```python
from build123d import *

# Parameters (mm, degrees)
F1_DEPTH = 73.66
F2_R     = 5.08


with BuildPart() as f1:
    # F0 (on Front) → F1 (new body)
    with BuildSketch(Plane.XZ):
        Polygon((-94.9451997876, 22.5552003831), (-94.9451997876, -16.4592005312), (-90.67799896, -16.4592005312), (-87.6299962401, -3.3528001513), (-65.6844004989, -3.3528001513), (-58.6740002036, -16.4592005312), (8.3820000291, -16.4592005312), (18.1356016546, -3.3528001513), (41.9100001454, -3.3528001513), (54.406799376, -16.4592005312), (69.6468055248, -16.4592005312), (62.3316019773, 16.1543991417), (23.3171992004, 16.1543991417), (-6.2483996153, 35.6616005301), (-55.3212016821, 35.6616005301), (-77.8764039278, 16.1543991417), (-87.9347994924, 16.1543991417), align=None)
    extrude(amount=F1_DEPTH)

    # F2
    f2_edges = [f1.edges().sort_by_distance(p)[0] for p in [
        (65.989204, 0, -0.152401),
        (62.331602, -36.83, 16.154399),
        (65.989204, -73.66, -0.152401),
        (42.824401, 0, 16.154399),
        (8.5344, 0, 25.908),
        (-6.2484, -36.83, 35.661601),
        (8.5344, -73.66, 25.908),
        (42.824401, -73.66, 16.154399),
        (23.317199, -36.83, 16.154399),
        (-30.784801, 0, 35.661601),
        (-55.321202, -36.83, 35.661601),
        (-30.784801, -73.66, 35.661601),
        (-66.598803, -73.66, 25.908),
        (-77.876404, -36.83, 16.154399),
        (-66.598803, 0, 25.908),
        (-82.905602, 0, 16.154399),
        (-87.934799, -36.83, 16.154399),
        (-89.153998, -73.66, -9.906),
        (-76.657198, -73.66, -3.3528),
        (-62.1792, -73.66, -9.906),
        (-25.146, -73.66, -16.459201),
        (13.258801, -73.66, -9.906),
        (30.022801, -73.66, -3.3528),
        (48.1584, -73.66, -9.906),
        (-82.905602, -73.66, 16.154399),
        (-91.44, 0, 19.3548),
        (-91.44, -73.66, 19.3548),
    ]]
    fillet(f2_edges, radius=F2_R)


solid = f1.part
```
Input: part model. Units: mm. Frame: model coordinates. A direction names the side the tool comes from. Give positions to 0.01 mm unless a question says otherwise; leave off trailing zeros. Order: outer loops, then holes, each group sorted by start corner. A loop starts at its lowest first (then second) coordinate and runs counter-clockwise, first axis right, second up.
1. Reachability of faces 1 (the cylindrical face through (-90.65, -72.13, -9.96)), 2 (the cylindrical face through (-92.187, -71.448, 18.836)), 3 (the flat face through (-62.23, -33.81, -9.81)), 4 (the flat face through (42, -36, 16.154)) from +Z, -Z, +X, -X, +Y, -Y: full face, straight path, thin tool, end or side. Return the list, or none.
Derived:
face 1: -Z, -Y
face 2: +Z, -Y
face 3: -Z, +Y, -Y
face 4: +Z, +X, +Y, -Y
2. Material intervals for L1, parallel to X at y = -12, z = -4; L2, parallel to X at y = -10.5, z = -10.5; L3, parallel to Z at x = -82.5, y = -27.5, sorted ascending.
Derived:
L1: x = -94.95 to -87.78, -65.34 to 17.65, 42.53 to 66.85
L2: x = -94.95 to -89.29, -61.86 to 12.82, 48.72 to 68.31
L3: z = -3.35 to 16.15
3. Pin query (flat end, axial travel): pin 1 (19 mm diameter, centred on x = 26.5, y = -18, fed in from -Z); pin 2 (1 mm diameter, centred on x = 18.5, z = 4.5, fed in from +Y); pin 3 (1.5 mm diameter, centred on x = 34.5, y = -17, fed in from +Z); pin 4 (1 mm diameter, centred on x = 41, y = -29, fed in from -Z). Return the tip coordinate at first contact, or that it passes through.
Derived:
pin 1: stops at z = -4.88
pin 2: stops at y = 0
pin 3: stops at z = 16.15
pin 4: stops at z = -3.35
4. Section B-B on x = 27. Return the cut outline in (y, z).
Derived:
outline: (-73.66, 1.73) arc R5.08 ccw to (-68.58, -3.35) - (0, -3.35) - (0, 11.07) arc R5.08 ccw to (-5.08, 16.15) - (-68.58, 16.15) arc R5.08 ccw to (-73.66, 11.07) - close
5. Section A-A on y = -36.5. Return the cut outline in (x, z).
Derived:
outline: (-94.95, -16.46) - (-90.68, -16.46) - (-87.63, -3.35) - (-65.68, -3.35) - (-58.67, -16.46) - (8.38, -16.46) - (18.14, -3.35) - (41.91, -3.35) - (54.41, -16.46) - (69.65, -16.46) - (63.22, 12.19) arc R5.08 ccw to (58.26, 16.15) - (24.84, 16.15) arc R5.08 cw to (22.04, 16.99) - (-4.98, 34.82) arc R5.08 ccw to (-7.77, 35.66) - (-53.43, 35.66) arc R5.08 ccw to (-56.75, 34.42) - (-76.45, 17.39) arc R5.08 cw to (-79.77, 16.15) - (-85.96, 16.15) arc R5.08 cw to (-89.39, 17.48) - (-94.95, 22.56) - close
